Input: part model. Units: mm. Frame: model coordinates. A direction names the side the tool comes from. Round coordinates to 2 decimals unless told otherwise and drop trailing zeros. Loops run counter-clockwise (first coordinate to the right, second up) from the corner with the lowest first, then second, coordinate; pieces in that order, holes last. Notation, with made-up numbers: (-39, 89.25) -> (-26, 89.25) arc R19 cw to (-26, 105.25) -> close; hole circle Ø7 at (24.5, -36). An arc over 180 degrees is marked (long way). Answer in a Markdown table with one row per item. Add a question column.
Q1. Mould query, pull axis Y, two halves, no side actions, for faces 3 (the face through (0, 0, 0)), 4 (the face through (0, -8, 2)), 5 (the face through (-12.13, 0.19, 1.51)). Classes: pulls with the +Y half, pulls with the -Y half, needs draft (parallel to the pull), parting line crosses it, or undercut.
Q2. Reachability of faces 1 (the face through (16.898, 0.176, 2.465)), 2 (the face through (-7, -4, 1)) from +Z, -Z, +X, -X, +Y, -Y: full face, straight path, thin tool, end or side. Return the list, or none.
Q3. Section C-C, the plane x = 10.4. Output: boundary loops of the cut face in (y, z) (3 decimals), and give its area (3 significant figures).
Q4. Section B-B, the plane z = 2.45. Give the number of separate pieces and of enclosed holes in the cut face, and give its area (3 significant figures).
Q5. Section A-A, the plane x = -7.7. Output: boundary loops of the cut face in (y, z) (3 decimals).
Q6. Ray query, L1, parallel to X at y = -0.25, z = 2.65; L2, parallel to Y at x = 11.9, z = 1.95 (3 decimals); L3, parallel to Y at x = -6, z = 4.2. Return the intervals inside material, ascending. Write a range as from..to.
Q7. Pin query (flat end, axial travel): pin 1 (5.5 mm diameter, centred on x = -10, y = 1.5, fed in from +Z); pin 2 (3 mm diameter, centred on y = 3.5, z = 1.5, fed in from +X); pin 3 (3 mm diameter, centred on x = -11, z = 3.5, fed in from +Y). Return the tip coordinate at first contact, or that it passes through.
```python
from build123d import *

# Parameters (mm, degrees)
BOSS_EXTRUDE1_DEPTH = 5
SKETCH2_R           = 3.9
CUT_EXTRUDE1_DEPTH  = 5
SKETCH3_R           = 4.435
CUT_EXTRUDE2_DEPTH  = 4
SKETCH4_R           = 4.75
CUT_EXTRUDE3_DEPTH  = 3
SKETCH5_R           = 5
CUT_EXTRUDE4_DEPTH  = 2
SKETCH6_R           = 5.6
CUT_EXTRUDE5_DEPTH  = 1
SKETCH7_R           = 0.375
CUT_EXTRUDE6_DEPTH  = 6


with BuildPart() as part:
    # Sketch1 → Boss-Extrude1 (new body)
    with BuildSketch(Plane.XY):
        with BuildLine():
            Line((-8.9, 8), (8.9, 8))
            ThreePointArc((8.9, 8), (16.9, 0), (8.9, -8))
            Line((8.9, -8), (-8.9, -8))
            ThreePointArc((-8.9, -8), (-16.9, 0), (-8.9, 8))
        make_face()
    extrude(amount=BOSS_EXTRUDE1_DEPTH)

    # Sketch2 → Cut-Extrude1 (cut)
    with BuildSketch(Plane.XY.offset(5)):
        with Locations((-7.7, 0)):
            Circle(SKETCH2_R)
    extrude(amount=-CUT_EXTRUDE1_DEPTH, mode=Mode.SUBTRACT)

    # Sketch3 → Cut-Extrude2 (cut)
    with BuildSketch(Plane.XY.offset(5)):
        with Locations((-7.7, 0)):
            Circle(SKETCH3_R)
    extrude(amount=-CUT_EXTRUDE2_DEPTH, mode=Mode.SUBTRACT)

    # Sketch4 → Cut-Extrude3 (cut)
    with BuildSketch(Plane.XY.offset(5)):
        with Locations((-7.7, 0)):
            Circle(SKETCH4_R)
    extrude(amount=-CUT_EXTRUDE3_DEPTH, mode=Mode.SUBTRACT)

    # Sketch5 → Cut-Extrude4 (cut)
    with BuildSketch(Plane.XY.offset(5)):
        with Locations((-7.7, 0)):
            Circle(SKETCH5_R)
    extrude(amount=-CUT_EXTRUDE4_DEPTH, mode=Mode.SUBTRACT)

    # Sketch6 → Cut-Extrude5 (cut)
    with BuildSketch(Plane.XY.offset(5)):
        with Locations((-7.7, 0)):
            Circle(SKETCH6_R)
    extrude(amount=-CUT_EXTRUDE5_DEPTH, mode=Mode.SUBTRACT)

    # Sketch7 → Cut-Extrude6 (cut, through all)
    with BuildSketch(Plane.XY.offset(5)):
        with Locations((10.4, 0)):
            Circle(SKETCH7_R)
        with Locations((8.9, 0)):
            Circle(SKETCH7_R)
        with Locations((11.9, 0)):
            Circle(SKETCH7_R)
        with Locations((8.9, -1.5)):
            Circle(SKETCH7_R)
        with Locations((10.4, -1.5)):
            Circle(SKETCH7_R)
        with Locations((11.9, -1.5)):
            Circle(SKETCH7_R)
        with Locations((8.9, 1.5)):
            Circle(SKETCH7_R)
        with Locations((10.4, 1.5)):
            Circle(SKETCH7_R)
        with Locations((11.9, 1.5)):
            Circle(SKETCH7_R)
    extrude(amount=-CUT_EXTRUDE6_DEPTH, mode=Mode.SUBTRACT)


solid = part.part
```
Answer block:
| question | item | result |
|---|---|---|
| 1 | face 3 | needs draft |
| 1 | face 4 | pulls with the -Y half |
| 1 | face 5 | undercut |
| 2 | face 1 | +Z, -Z, +X |
| 2 | face 2 | +Z |
| 3 | outline | (-7.858, 0) -> (-1.875, 0) -> (-1.875, 5) -> (-7.858, 5) -> close; (-1.125, 0) -> (-0.375, 0) -> (-0.375, 5) -> (-1.125, 5) -> close; (0.375, 0) -> (1.125, 0) -> (1.125, 5) -> (0.375, 5) -> close; (1.875, 0) -> (7.858, 0) -> (7.858, 5) -> (1.875, 5) -> close |
| 3 | area | 67.3 mm^2 |
| 4 | separate pieces | 1 |
| 4 | enclosed holes | 10 |
| 4 | area | 411 mm^2 |
| 5 | outline | (-8, 0) -> (-3.9, 0) -> (-3.9, 1) -> (-4.435, 1) -> (-4.435, 2) -> (-4.75, 2) -> (-4.75, 3) -> (-5, 3) -> (-5, 4) -> (-5.6, 4) -> (-5.6, 5) -> (-8, 5) -> close; (3.9, 0) -> (8, 0) -> (8, 5) -> (5.6, 5) -> (5.6, 4) -> (5, 4) -> (5, 3) -> (4.75, 3) -> (4.75, 2) -> (4.435, 2) -> (4.435, 1) -> (3.9, 1) -> close |
| 6 | L1 | -16.9..-12.44, -2.96..8.62, 9.18..10.12, 10.68..11.62, 12.18..16.9 |
| 6 | L2 | -7.416..-1.875, -1.125..-0.375, 0.375..1.125, 1.875..7.416 |
| 6 | L3 | -8..-5.34, 5.34..8 |
| 7 | pin 1 | z = 4 |
| 7 | pin 2 | x = 16.65 |
| 7 | pin 3 | y = 7.98 |
